Input: part model. Units: mm. Frame: model coordinates. A direction names the side the tool comes from. Coordinates: 2 decimals unless noted, no trailing zeros. Order: outer loops, then holes, each group sorted by start corner. A loop starts at its lowest first (then second) coordinate and runs counter-clockwise, first axis right, second up. Notation, with made-up numbers: M 6.25,76.25 L 55.25,76.25 A33 cw 55.25,110.25 Z; hole C -14,41 d11. An arc over 180 degrees is marked long. One line per item, written item: value.
```python
from build123d import *

# Parameters (mm, degrees)
F1_DEPTH = 11.5
F2_R     = 1.75
F3_DEPTH = 25
F4_R     = 1


with BuildPart() as f1:
    # F0 (on Top) → F1 (new body)
    with BuildSketch(Plane.XY):
        with BuildLine():
            ThreePointArc((0, 0.8), (5.13633, 0.906445), (10.25, 1.4))
            Line((10.25, 1.4), (17.584028, 0.051845))
            ThreePointArc((17.584028, 0.051845), (21.307427, 0.828514), (23.407092, 4))
            ThreePointArc((23.407092, 4), (20.608046, 1.678425), (16.976419, 1.867262))
            Line((16.976419, 1.867262), (11.75, 2.712208))
            Line((11.75, 2.712208), (11.75, 7.455321))
            ThreePointArc((11.75, 7.455321), (5.882541, 7.915111), (0, 8.1))
            ThreePointArc((0, 8.1), (-5.882541, 7.915111), (-11.75, 7.455321))
            Line((-11.75, 7.455321), (-11.75, 2.712208))
            Line((-11.75, 2.712208), (-16.976419, 1.867262))
            ThreePointArc((-16.976419, 1.867262), (-20.608046, 1.678425), (-23.407092, 4))
            ThreePointArc((-23.407092, 4), (-21.307427, 0.828514), (-17.584028, 0.051845))
            Line((-17.584028, 0.051845), (-10.25, 1.4))
            ThreePointArc((-10.25, 1.4), (-5.13633, 0.906445), (0, 0.8))
        make_face()
        Polygon((10.25, 5.8), (10.25, 3), (0, 3), (-10.25, 3), (-10.25, 5.8), (0, 5.8), align=None, mode=Mode.SUBTRACT)
    extrude(amount=F1_DEPTH)

    # F2 (on Front) → F3 (cut)
    with BuildSketch(Plane.XZ):
        with Locations((0, 5.75)):
            Circle(F2_R)
    extrude(amount=-F3_DEPTH, mode=Mode.SUBTRACT)

    # F4
    f4_edges = [f1.edges().sort_by_distance(p)[0] for p in [
        (-11.75, 7.455321, 5.75),
        (11.75, 7.455321, 5.75),
    ]]
    fillet(f4_edges, radius=F4_R)


solid = f1.part
```
(1) Cut plane A-A on y = 4.5. Output: boundary loops of the cut face in (x, z), plus the area to 3 significant figures.
Data:
outline: M -11.75,0 L -10.25,0 L -10.25,11.5 L -11.75,11.5 Z; M 10.25,0 L 11.75,0 L 11.75,11.5 L 10.25,11.5 Z
area: 34.5 mm2
(2) Cut plane D-D on z = 5.75. Output: boundary loops of the cut face in (x, y), plus the area to 3 significant figures.
Data:
outline: M -23.41,4 A5 ccw -17.58,0.05 L -10.25,1.4 A68.06 ccw -1.75,0.79 L -1.75,3 L -10.25,3 L -10.25,5.8 L -1.75,5.8 L -1.75,8.07 A125.81 ccw -10.84,7.54 A1 ccw -11.75,6.55 L -11.75,2.71 L -16.98,1.87 A5 cw Z; M 1.75,0.79 A68.06 ccw 10.25,1.4 L 17.58,0.05 A5 ccw 23.41,4 A5 cw 16.98,1.87 L 11.75,2.71 L 11.75,6.55 A1 ccw 10.84,7.54 A125.81 ccw 1.75,8.07 L 1.75,5.8 L 10.25,5.8 L 10.25,3 L 1.75,3 Z
area: 121 mm2
(3) Access query for faces 1 (the cylindrical face through (-5.21, 0.91, 5.67)), 2 (the flat face through (11.75, 5, 6)), 3 (the flat face through (2, 3, 6)). Directions: +Z, -Z, +X, -X, +Y, -Y. A direction counts if a zero-diameter tool reaches every point of the face in a straight line with its end or side. Return the directions, or none.
Data:
face 1: +Z, -Z, -Y
face 2: +Z, -Z, +Y
face 3: +Z, -Z
(4) Ray query, line 1 (Z direction, x = 0, y = 1.9); line 2 (X direction, y = 5, z = 6.5); line 3 (Y direction, x = -9, z = 3.5). Return the intervals inside material, ascending. Write a range as from..to.
Data:
line 1: z = 0..4, 7.5..11.5
line 2: x = -11.75..-10.25, 10.25..11.75
line 3: y = 1.24..3, 5.8..7.71
(5) First-contact query: pin 1 (6 mm diameter, centred on x = 1.5, z = 9, fed in from -Y); pin 2 (1.5 mm diameter, centred on y = 2.5, z = 5, fed in from +X); pin 3 (1.4 mm diameter, centred on y = 5, z = 3.5, fed in from -X). Flat tips, straight axial feed; report the tip coordinate or a pass-through.
Data:
pin 1: stops at y = 0.79
pin 2: stops at x = 23.2
pin 3: stops at x = -11.75
(6) Cut plane B-B on z = 3.25. Output: boundary loops of the cut face in (x, y), plus the area to 3 significant figures.
Data:
outline: M -23.41,4 A5 ccw -17.58,0.05 L -10.25,1.4 A68.06 ccw 0,0.8 A68.06 ccw 10.25,1.4 L 17.58,0.05 A5 ccw 23.41,4 A5 cw 16.98,1.87 L 11.75,2.71 L 11.75,6.55 A1 ccw 10.84,7.54 A125.81 ccw 0,8.1 A125.81 ccw -10.84,7.54 A1 ccw -11.75,6.55 L -11.75,2.71 L -16.98,1.87 A5 cw Z; hole M -10.25,3 L 10.25,3 L 10.25,5.8 L -10.25,5.8 Z
area: 136 mm2
(7) Draft query along Z for faces 4 (the cylindrical face through (0, 7, 4)), 5 (the flat face through (0, 2, 11.5)), 6 (the flat face through (-14.3, 2.3, 5.7)). Return one class per face: released by +Z, released by -Z, zero draft, split by the parting line, or undercut.
Data:
face 4: undercut
face 5: released by +Z
face 6: zero draft
(8) Cut plane C-C on x = -6. Output: boundary loops of the cut face in (y, z), plus the area to 3 significant figures.
Data:
outline: M 0.96,0 L 3,0 L 3,11.5 L 0.96,11.5 Z; M 5.8,0 L 7.91,0 L 7.91,11.5 L 5.8,11.5 Z
area: 47.7 mm2
